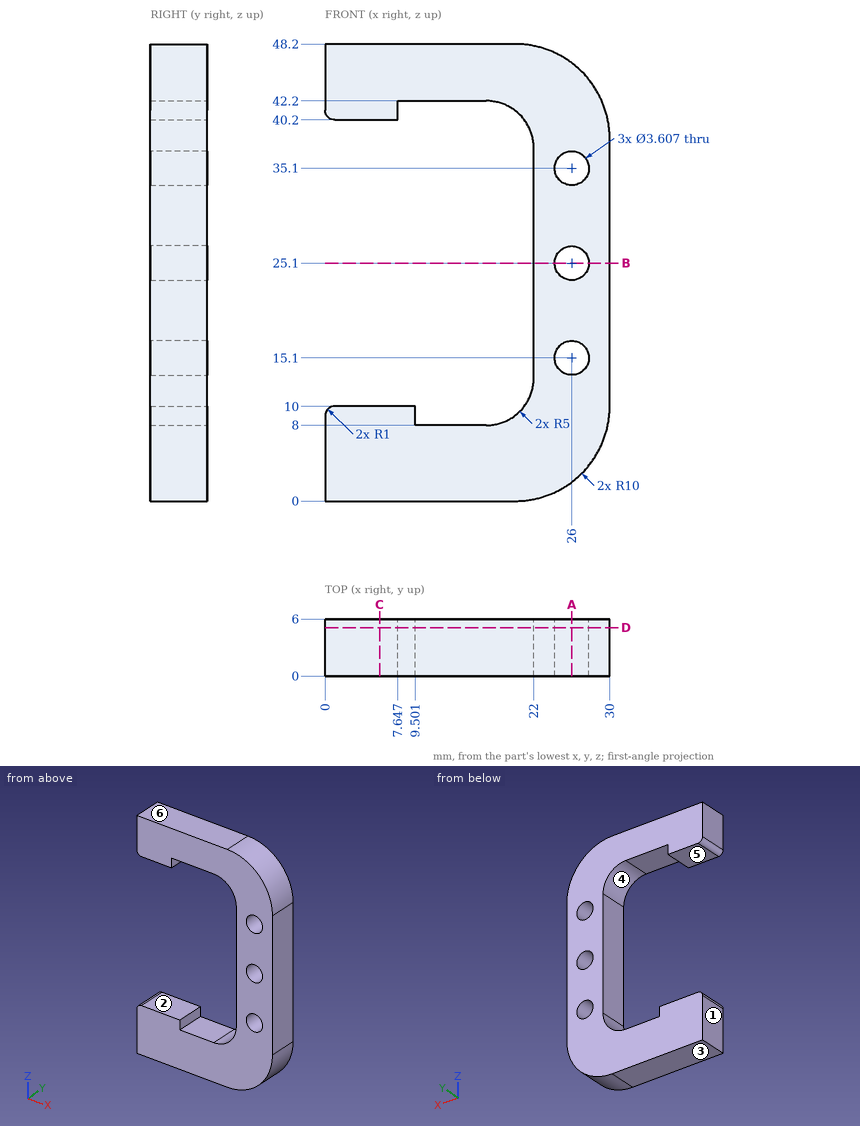
Geometry: see drawing. Coordinates: mm, zero at the bounding-box minimum. A direction names the side the tool comes from. Give positions to 0.01 mm unless a question says otherwise; leave off trailing zeros. Loops run counter-clockwise (first coordinate to the right, second up) from the corner with the lowest first, then second, coordinate; pieces in that order, holes last. Notation, with made-up numbers: (67, 10.25) -> (92, 10.25) arc R26 cw to (92, 29.25) -> close; hole circle Ø2 at (-30, 17). An arc over 180 degrees is marked (long way). Answer as a JSON object with one key per item and string values. Group by question number.
Item 1: Line query: probe 1 along X at (y, z) = (3.05, 25.1); probe 2 along Z at (x, y) = (13, 3.25); probe 3 along Z at (x, y) = (26.25, 1.55) (1 decimal). Output: solid intervals per line, ascending.
Item 2: Pin query (flat end, axial travel): P1, Ø1.6, axis at y = 3.5, z = 9, coming from the +X side; P2, Ø0.6, axis at y = 2.5, z = 41.5, coming from the +X side; P3, Ø1.5, axis at x = 26.5, y = 2.5, coming from the +Z side. Return the tip coordinate at first contact, or that it passes through.
Item 3: Cut plane C-C, the plane x = 5.75. Return the cut outline in (y, z).
Item 4: Cut plane B-B, the plane z = 25.1. Return the cut outline in (x, y).
Item 5: Cut plane A-A, the plane x = 26. Return the cut outline in (y, z).
Item 6: Cut plane D-D, the plane y = 5.1. Return the cut outline in (x, z).
Item 7: Reachability of the marked faces 4, 5 and 6 from +Z, -Z, +X, -X, +Y, -Y: full face, straight path, thin tool, end or side. Return the list, or none.
Item 8: Pull-direction query (Z, two-part tool) for the marked faces 1, 2 and 3; classes: released by +Z, released by -Z, zero draft, split by the parting line, or undercut.
Checks:
{
 "1": {"probe 1": "x = 22 to 24.2, 27.8 to 30", "probe 2": "z = 0 to 8, 42.2 to 48.2", "probe 3": "z = 2.2 to 13.3, 16.9 to 23.3, 26.9 to 33.3, 36.9 to 46"},
 "2": {"P1": "stops at x = 30", "P2": "stops at x = 29.54", "P3": "stops at z = 46.38"},
 "3": {"outline": "(0, 0) -> (6, 0) -> (6, 10) -> (0, 10) -> close; (0, 40.2) -> (6, 40.2) -> (6, 48.2) -> (0, 48.2) -> close"},
 "4": {"outline": "(22, 0) -> (24.2, 0) -> (24.2, 6) -> (22, 6) -> close; (27.8, 0) -> (30, 0) -> (30, 6) -> (27.8, 6) -> close"},
 "5": {"outline": "(0, 2) -> (6, 2) -> (6, 13.3) -> (0, 13.3) -> close; (0, 16.9) -> (6, 16.9) -> (6, 23.3) -> (0, 23.3) -> close; (0, 26.9) -> (6, 26.9) -> (6, 33.3) -> (0, 33.3) -> close; (0, 36.9) -> (6, 36.9) -> (6, 46.2) -> (0, 46.2) -> close"},
 "6": {"outline": "(0, 0) -> (20, 0) arc R10 ccw to (30, 10) -> (30, 38.2) arc R10 ccw to (20, 48.2) -> (0, 48.2) -> (0, 41.2) arc R1 ccw to (1, 40.2) -> (7.65, 40.2) -> (7.65, 42.2) -> (17, 42.2) arc R5 cw to (22, 37.2) -> (22, 13) arc R5 cw to (17, 8) -> (9.5, 8) -> (9.5, 10) -> (1, 10) arc R1 ccw to (0, 9) -> close; hole circle Ø3.61 at (26, 15.1); hole circle Ø3.61 at (26, 25.1); hole circle Ø3.61 at (26, 35.1)"},
 "7": {"face 4": "+Y, -Y", "face 5": "-X, +Y, -Y", "face 6": "+Z, +X, -X, +Y, -Y"},
 "8": {"face 1": "zero draft", "face 2": "undercut", "face 3": "released by -Z"}
}
